The listing builds one solid part. Answer for the finished solid, in the listing's coordinates (mm). A direction names the side the tool comes from. Coordinates: 2 decimals unless noted, no trailing zeros. Write each loop counter-clockwise with the first axis right and the second up, starting at its lowest first coordinate (ties: lowest second). Pieces come first, ordered by that corner, then holes.
from build123d import *

# Parameters (mm, degrees)
EXTRUDE_1_DEPTH     = 14
SKETCH_3_R          = 3.7
CUT_EXTRUDE_1_DEPTH = 19
SKETCH_5_R          = 4.3
CUT_EXTRUDE_2_DEPTH = 0.8
SKETCH_6_R          = 4.3
CUT_EXTRUDE_3_DEPTH = 0.8
SKETCH_8_W          = 40
SKETCH_8_H          = 14
CUT_EXTRUDE_4_DEPTH = 12
SKETCH_9_W          = 2.5
SKETCH_9_H          = 5
CUT_EXTRUDE_5_DEPTH = 5
CUT_EXTRUDE_6_DEPTH = 5
EXTRUDE_3_DEPTH     = 6
EXTRUDE_5_DEPTH     = 14
FILLET_5_R          = 0.25
SKETCH_15_R         = 1
CUT_EXTRUDE_7_DEPTH = 14


with BuildPart() as part:
    # 스케치1 → 보스-돌출1 (new body)
    with BuildSketch(Plane(origin=(0, 0, 0), x_dir=(1, 0, 0), z_dir=(0, 1, 0))):
        with BuildLine():
            Line((0, 8.5), (80, 8.5))
            ThreePointArc((80, 8.5), (88.5, 0), (80, -8.5))
            Line((80, -8.5), (0, -8.5))
            ThreePointArc((0, -8.5), (-8.5, 0), (0, 8.5))
        make_face()
    extrude(amount=EXTRUDE_1_DEPTH)

    # 스케치2 → 회전1 (revolve)
    with BuildSketch(Plane(origin=(0, 0, 0), x_dir=(0, 0, -1), z_dir=(1, 0, 0))):
        Polygon((0, 14), (0, 16.5), (8.5, 16.5), (7.15, 15.25), (8.5, 14), align=None)
        Polygon((0, 0), (0, -2.5), (8.5, -2.5), (7.15, -1.25), (8.5, 0), align=None)
    revolve(axis=Axis((0, 14, 0), (0, -1, 0)))

    # 스케치3 → 컷-돌출1 (cut)
    with BuildSketch(Plane(origin=(0, 16.5, 0), x_dir=(1, 0, 0), z_dir=(0, 1, 0))):
        Circle(SKETCH_3_R)
    extrude(amount=-CUT_EXTRUDE_1_DEPTH, mode=Mode.SUBTRACT)

    # 스케치5 → 컷-돌출2 (cut)
    with BuildSketch(Plane(origin=(0, 16.5, 0), x_dir=(1, 0, 0), z_dir=(0, 1, 0))):
        Circle(SKETCH_5_R)
    extrude(amount=-CUT_EXTRUDE_2_DEPTH, mode=Mode.SUBTRACT)

    # 스케치6 → 컷-돌출3 (cut)
    with BuildSketch(Plane.XZ.offset(2.5)):
        Circle(SKETCH_6_R)
    extrude(amount=-CUT_EXTRUDE_3_DEPTH, mode=Mode.SUBTRACT)

    # 스케치8 → 컷-돌출4 (cut)
    with BuildSketch(Plane.XY.offset(8.5)):
        with Locations((60, 7)):
            Rectangle(SKETCH_8_W, SKETCH_8_H)
    extrude(amount=-CUT_EXTRUDE_4_DEPTH, mode=Mode.SUBTRACT)

    # 스케치9 → 컷-돌출5 (cut)
    with BuildSketch(Plane.XY.offset(-3.5)):
        with Locations((46.25, 7)):
            Rectangle(SKETCH_9_W, SKETCH_9_H)
    extrude(amount=-CUT_EXTRUDE_5_DEPTH, mode=Mode.SUBTRACT)

    # 스케치11 → 컷-돌출6 (cut)
    with BuildSketch(Plane(origin=(0, 4.5, 0), x_dir=(1, 0, 0), z_dir=(0, 1, 0))):
        Polygon((47.5, 3.5), (52.5, 3.5), (47.5, 8.5), (40, 8.5), (45, 3.5), align=None)
    extrude(amount=CUT_EXTRUDE_6_DEPTH, mode=Mode.SUBTRACT)

    # 스케치12 → 보스-돌출3 (add)
    with BuildSketch(Plane.XY.offset(-3.5)):
        Polygon((80, 14), (70, 14), (70, 10.75), (77, 10.75), (77, 3.25), (70, 3.25), (70, 0), (80, 0), align=None)
        Polygon((50, 14), (50, 10.75), (43, 10.75), (43, 3.25), (50, 3.25), (50, 0), (40, 0), (40, 14), align=None)
    extrude(amount=EXTRUDE_3_DEPTH)

    # 스케치14 → 보스-돌출5 (add)
    with BuildSketch(Plane.XZ):
        Polygon((40, 8.5), (40.5, 8.5), (40, 7.5), align=None)
        Polygon((80, 8.5), (79.5, 8.5), (80, 7.5), align=None)
    extrude(amount=-EXTRUDE_5_DEPTH)

    # 필렛5
    fillet_5_edges = [part.edges().sort_by_distance(p)[0] for p in [
        (40.5, 7, 8.5),
        (79.5, 7, 8.5),
    ]]
    fillet(fillet_5_edges, radius=FILLET_5_R)

    # 스케치15 → 컷-돌출7 (cut)
    with BuildSketch(Plane(origin=(0, 14, 0), x_dir=(1, 0, 0), z_dir=(0, 1, 0))):
        with Locations((15, 0)):
            Circle(SKETCH_15_R)
    extrude(amount=-CUT_EXTRUDE_7_DEPTH, mode=Mode.SUBTRACT)


solid = part.part
Q1. Determine the mould class of faces 1 (the face through (2, -2.5, -4)), 2 (the face through (16, 7, 0)) for opening direction X: released by +X, released by -X, zero draft, split by the parting line, or undercut.
Answers below:
face 1: zero draft
face 2: undercut
Q2. Find the intervals of material crossed by probe 1 along X at (y, z) = (11.25, 0); probe 2 along X at (y, z) = (8.5, 0); probe 3 along Y at (x, z) = (47.5, -3), in increasing order.
Answers below:
probe 1: x = -8.5 to -3.7, 3.7 to 14, 16 to 50, 70 to 88.5
probe 2: x = -8.5 to -3.7, 3.7 to 14, 16 to 43, 77 to 88.5
probe 3: y = 0 to 3.25, 10.75 to 14
Q3. The part is cut by section D-D, the plane x = 60. Write down the section's boundary in (y, z).
Answers below:
outline: (0, -8.5) - (14, -8.5) - (14, -3.5) - (0, -3.5) - close
Q4. The part is cut by section C-C, the plane x = 78.5. Write down the section's boundary in (y, z), then the cut area to 3 significant figures.
Answers below:
outline: (0, -8.5) - (14, -8.5) - (14, 2.5) - (0, 2.5) - close
area: 154 mm2
Q5. The part is cut by section B-B, the plane z = 0. State how many separate pieces and enclosed holes the cut face has, then the cut area to 3 significant figures.
Answers below:
separate pieces: 4
enclosed holes: 0
area: 881 mm2
Q6. Which of the six approach directions +Z, -Z, +X, -X, +Y, -Y give full straight-line access (tool end or side, diameter ignored) to faces 3 (the face through (74, 3.25, -1)), 4 (the face through (-4.296, -2.106, 0.189)), 5 (the face through (40, 7, 5))?
Answers below:
face 3: +Z
face 4: -Y
face 5: +Y, -Y
Q7. The part is cut by section A-A, the plane x = 15. Write down the section's boundary in (y, z).
Answers below:
outline: (0, -8.5) - (14, -8.5) - (14, -1) - (0, -1) - close; (0, 1) - (14, 1) - (14, 8.5) - (0, 8.5) - close
Q8. Given pin 1 (8 mm diameter, centred on x = 78, z = -5.5, fed in from +Y); pin 2 (7 mm diameter, centred on x = 0, z = 0, fed in from -Y) (3 decimals); pin 3 (5 mm diameter, centred on x = 29, z = 1, fed in from -Y); pin 4 (5.5 mm diameter, centred on y = 6.5, z = 5, fed in from -X), each flat-ended and moving along its own axis, determine where each tip first touches the part or whether it passes through.
Answers below:
pin 1: stops at y = 14
pin 2: passes through
pin 3: stops at y = 0
pin 4: stops at x = -8.2
